Verification items for the finished model (mm, model axes). Face numbers are marked on the shaded views. Round coordinates to 2 decimals unless told otherwise and drop trailing zeros. Loops run counter-clockwise (first coordinate to the right, second up) from the corner with the lowest first, then second, coordinate; pieces in that order, holes last. Notation, with made-up numbers: (49.5, -14.5) -> (97.5, -14.5) arc R21 ccw to (97.5, 10.5) -> close; hole circle Ø3 at (13, -14). An arc over 180 degrees is marked (long way). Write item = value, one per line.
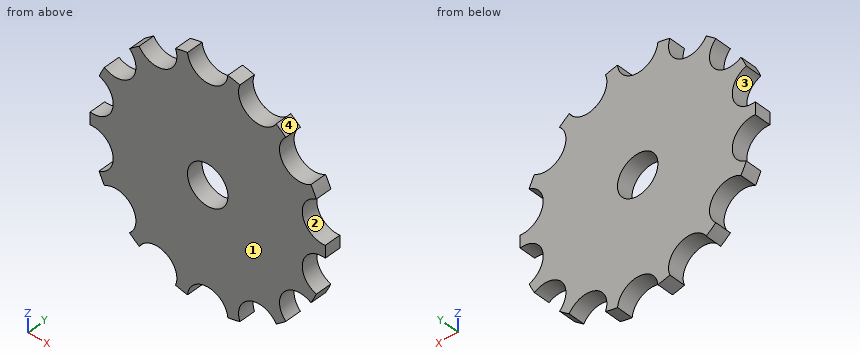
Solid Edge part; units mm, degrees
sketch "Sketch1" plane through (0, 0, 0) normal (0, -1, 0) x (1, 0, 0)
  circle A0 centre (0, 0) radius 14.545
extrude "Protrusion1" add sketch "Sketch1" along normal mid plane 2
hole "Hole_16" at (0, 1, 14.545) direction (0, -1, 0) diameter 5 end up to next
pattern_circular "Pattern_2" count 14 over 360 about axis through (0, 1, 0) along (0, -1, 0) of "Hole_16"
hole "Hole_30" at (0, -1, 0) direction (0, 1, 0) diameter 5 end up to next
(1) Material ranges on probe 1 along X at (y, z) = (0.55, 0) (3 decimals); probe 2 along Z at (x, y) = (0, -0.2) (3 decimals); probe 3 along Z at (x, y) = (12, -0.05), recorded low to high. Write a range as from..to.
Filled sheet:
probe_1 = -14.545..-2.5, 2.5..14.545
probe_2 = -12.045..-2.5, 2.5..12.045
probe_3 = -6.65..-4.46, -2.01..2.01, 4.46..6.65
(2) Draft check along Z on the marked faces 1, 2, 3 and 4. Enter one of: released by +Z, released by -Z, zero draft, split by the parting line, or undercut.
Filled sheet:
face_1 = zero draft
face_2 = undercut
face_3 = undercut
face_4 = released by +Z
(3) Sectioned sample at D-D, the plane z = 3. Record the cut outline in (x, y).
Filled sheet:
outline = (-11.69, -1) -> (11.69, -1) -> (11.69, 1) -> (-11.69, 1) -> close
(4) Go/stop test with a flat-tipped pin: pin 1 Ø1 at (y, z) = (0.5, 4.5) entering from +X. Record where the tip stops, or that it passes through.
Filled sheet:
pin_1 = 12.41
(5) Sectioned sample at B-B, the plane x = 0. Record the cut outline in (y, z) (3 decimals), and give its area (3 significant figures).
Filled sheet:
outline = (-1, -12.045) -> (1, -12.045) -> (1, -2.5) -> (-1, -2.5) -> close; (-1, 2.5) -> (1, 2.5) -> (1, 12.045) -> (-1, 12.045) -> close
area = 38.2 mm2
(6) Sectioned sample at A-A, the plane z = 0. Record the cut outline in (x, y) (3 decimals).
Filled sheet:
outline = (-14.545, -1) -> (-2.5, -1) -> (-2.5, 1) -> (-14.545, 1) -> close; (2.5, -1) -> (14.545, -1) -> (14.545, 1) -> (2.5, 1) -> close
